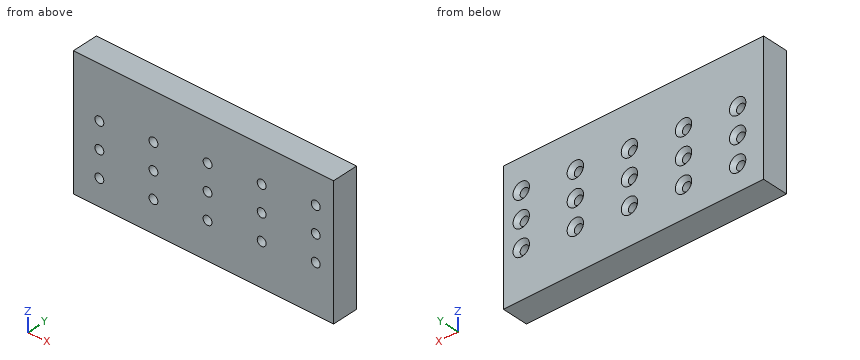
from build123d import *

# Parameters (mm, degrees)
SKETCH1_W                                       = 100
SKETCH1_H                                       = 50
BOSS_EXTRUDE1_DEPTH                             = 10
CSK_FOR_M3_FLAT_HEAD_MACHINE_SCREW1_D           = 3.4
CSK_FOR_M3_FLAT_HEAD_MACHINE_SCREW1_CSINK_D     = 6.3
CSK_FOR_M3_FLAT_HEAD_MACHINE_SCREW1_CSINK_ANGLE = 90
LPATTERN1_COUNT                                 = 5
LPATTERN1_PITCH                                 = 20.88337397
LPATTERN1_COUNT_DIR2                            = 3
LPATTERN1_PITCH_DIR2                            = 10


with BuildPart() as part:
    # Sketch1 → Boss-Extrude1 (new body)
    with BuildSketch(Plane(origin=(0, 0, 0), x_dir=(1, 0, 0), z_dir=(0, 1, 0))):
        Rectangle(SKETCH1_W, SKETCH1_H)
    extrude(amount=BOSS_EXTRUDE1_DEPTH)

    # CSK for M3 Flat Head Machine Screw1 (through all)
    with Locations(Plane(origin=(-40, 10, -15), x_dir=(0, 0, 1), z_dir=(0, 1, 0))):
        with Locations((0, 0)):
            csk_for_m3_flat_head_machine_screw1 = CounterSinkHole(CSK_FOR_M3_FLAT_HEAD_MACHINE_SCREW1_D / 2, CSK_FOR_M3_FLAT_HEAD_MACHINE_SCREW1_CSINK_D / 2, counter_sink_angle=CSK_FOR_M3_FLAT_HEAD_MACHINE_SCREW1_CSINK_ANGLE)

    # LPattern1: CSK for M3 Flat Head Machine Screw1 5 × 3
    with Locations(*[Vector(0.9950371902099892, 0, 0.099503719020999) * (i * LPATTERN1_PITCH) + Vector(0, 0, 1) * (j * LPATTERN1_PITCH_DIR2) for i in range(LPATTERN1_COUNT) for j in range(LPATTERN1_COUNT_DIR2) if (i, j) != (0, 0)]):
        add(csk_for_m3_flat_head_machine_screw1, mode=Mode.SUBTRACT)


solid = part.part
Design review of the part built by this model. Coordinates are the model's own, in mm. Give positions to 0.01 mm unless a question says otherwise; leave off trailing zeros. Order: outer loops, then holes, each group sorted by start corner. A loop starts at its lowest first (then second) coordinate and runs counter-clockwise, first axis right, second up. Notation, with made-up numbers: (53, 20) - (107, 20) arc R27 cw to (107, 38) - close; hole circle Ø10 at (23.5, 49). An arc over 180 degrees is marked (long way). Write item = value, one per line. Start each with the question number.
Q1. We need section B-B on y = 4.25. State how many separate pieces and enclosed holes the cut face has, plus the area to 3 significant figures.
Q2. Clearance check with flat-ended pins moving along their axes: pin 1 Ø4.5 at (x, z) = (43.12, 13.31) entering from +Y; pin 2 Ø5.5 at (x, z) = (-40, -15) entering from +Y; pin 3 Ø4 at (x, z) = (22.34, 11.23) entering from +Y; pin 4 Ø1 at (x, z) = (1.5, 10) entering from -Y. State where each tip first meets the part, or that it passes through.
Q3. We need section A-A on x = -40. State the section outline as (y, z) points.
Q4. To check wall thickness, follow L1, parallel to Z at x = -40, y = 4.5; L2, parallel to X at y = 7, z = -5.5; L3, parallel to X at y = 0.75, z = 10. State the ranges of each line that lie inside material, in increasing order. Write a range as from..to.
Working result:
q1.separate_pieces = 1
q1.enclosed_holes = 15
q1.area = 4,860 mm²
q2.pin_1 = 9.1
q2.pin_2 = 9.6
q2.pin_3 = 8.85
q2.pin_4 = through
q3.outline = (0, -25) - (10, -25) - (10, -18.15) - (8.55, -16.7) - (0, -16.7) - close; (0, -13.3) - (8.55, -13.3) - (10, -11.85) - (10, -8.15) - (8.55, -6.7) - (0, -6.7) - close; (0, -3.3) - (8.55, -3.3) - (10, -1.85) - (10, 1.85) - (8.55, 3.3) - (0, 3.3) - close; (0, 6.7) - (8.55, 6.7) - (10, 8.15) - (10, 25) - (0, 25) - close
q4.L1 = -25..-16.7, -13.3..-6.7, -3.3..3.3, 6.7..25
q4.L2 = -50..-41.62, -38.38..41.9, 44.33..50
q4.L3 = -50..0.08, 3.04..21.17, 23.51..50
